Here's how the part is built. I have some questions about the finished solid (model axes, mm). A direction names the side the tool comes from. Give positions to 0.01 mm unless a question says otherwise; leave off trailing zeros. Order: outer loops, then holes, each group sorted by start corner. A loop starts at its lowest first (then second) coordinate and runs counter-clockwise, first axis right, second up. Notation, with made-up numbers: M 28,-27 L 74,-27 A20 ccw 74,12 Z; hole C 16,2 d2. An arc over 180 degrees is marked long. Use one line per item in the form item = value.
from build123d import *

# Parameters (mm, degrees)
SKETCH_1_W      = 50
SKETCH_1_H      = 50
SKETCH_1_R      = 13
SKETCH_1_R_2    = 2
EXTRUDE_1_DEPTH = 2
SKETCH_2_W      = 50
SKETCH_2_H      = 50
SKETCH_2_R      = 12.5
SKETCH_2_R_2    = 2.5
EXTRUDE_2_DEPTH = 2
EXTRUDE_3_DEPTH = 2


with BuildPart() as part:
    # 草图1 → 凸台-拉伸1 (new body)
    with BuildSketch(Plane(origin=(0, 0, 0), x_dir=(1, 0, 0), z_dir=(0, 1, 0))):
        Rectangle(SKETCH_1_W, SKETCH_1_H)
        with Locations(Location((0, 3, 0), (0, 0, 270))):
            Circle(SKETCH_1_R, mode=Mode.SUBTRACT)
        with Locations(Location((0, 20.5, 0), (0, 0, 270))):
            Circle(SKETCH_1_R_2, mode=Mode.SUBTRACT)
        with Locations(Location((0, -14.5, 0), (0, 0, 270))):
            Circle(SKETCH_1_R_2, mode=Mode.SUBTRACT)
        with Locations(Location((17.5, 3, 0), (0, 0, 270))):
            Circle(SKETCH_1_R_2, mode=Mode.SUBTRACT)
        with Locations(Location((-17.5, 3, 0), (0, 0, 270))):
            Circle(SKETCH_1_R_2, mode=Mode.SUBTRACT)
    extrude(amount=EXTRUDE_1_DEPTH)

    # 草图2 → 凸台-拉伸2 (add)
    with BuildSketch(Plane.XY.offset(25)):
        with Locations((0, 25)):
            Rectangle(SKETCH_2_W, SKETCH_2_H)
        with Locations((0, 26)):
            Circle(SKETCH_2_R, mode=Mode.SUBTRACT)
        with Locations((-15, 41)):
            Circle(SKETCH_2_R_2, mode=Mode.SUBTRACT)
        with Locations((15, 41)):
            Circle(SKETCH_2_R_2, mode=Mode.SUBTRACT)
        with Locations((15, 11)):
            Circle(SKETCH_2_R_2, mode=Mode.SUBTRACT)
        with Locations((-15, 11)):
            Circle(SKETCH_2_R_2, mode=Mode.SUBTRACT)
    extrude(amount=-EXTRUDE_2_DEPTH)

    # 草图3 → 凸台-拉伸3 (add)
    with BuildSketch(Plane(origin=(25, 0, 0), x_dir=(0, 0, -1), z_dir=(1, 0, 0))):
        Polygon((-25, 0), (0, 0), (-25, 25), align=None)
    extrude_3 = extrude(amount=-EXTRUDE_3_DEPTH)

    # 镜向2: 凸台-拉伸3 across plane
    add(extrude_3.mirror(Plane(origin=(0, 0, 0), x_dir=(0, 0, 1), z_dir=(1, 0, 0))))


solid = part.part
Q1. I want a section at C-C on y = 26. Write out the boundary of the cut face in (x, z), then the cut area to 3 significant figures.
Found:
outline = M -25,23 L -12.5,23 L -12.5,25 L -25,25 Z; M 12.5,23 L 25,23 L 25,25 L 12.5,25 Z
area = 50.0 mm²
Q2. I'm going to push flat-ended pins straight in: pin 1 Ø6 at (x, y) = (-15, 11) entering from -Z; pin 2 Ø2.5 at (x, z) = (0, 14.5) entering from +Y; pin 3 Ø1 at (x, z) = (19.5, 5) entering from +Y. Where does each tip first touch, or does it pass through?
Found:
pin_1 = 23
pin_2 = through
pin_3 = 2
Q3. Thinking about a two-plate mould opening in Z: for faces 1 (the face through (3.9, 1, 9.4)), 2 (the face through (24, 12, 12)), 3 (the face through (23, 8, 17)), which applies, +Z half, -Z half, draft (parallel to the pull), parting line (faces both ways), or undercut?
Found:
face_1 = undercut
face_2 = -Z half
face_3 = draft
Q4. I want a section at D-D on x = 0. Write out the boundary of the cut face in (y, z), then the cut area to 3 significant figures.
Found:
outline = M 0,-25 L 2,-25 L 2,-22.5 L 0,-22.5 Z; M 0,-18.5 L 2,-18.5 L 2,-16 L 0,-16 Z; M 0,10 L 2,10 L 2,12.5 L 0,12.5 Z; M 0,16.5 L 2,16.5 L 2,23 L 13.5,23 L 13.5,25 L 0,25 Z; M 38.5,23 L 50,23 L 50,25 L 38.5,25 Z
area = 78.0 mm²
Q5. I need wall thicknesses on L1, parallel to Y at x = -15, z = 24; L2, parallel to X at y = 8.5, z = 13; L3, parallel to Y at x = -10, z = -18.5. Which ranges of each line are inside material? Lowest first, please.
Found:
L1 = 0 to 8.5, 13.5 to 38.5, 43.5 to 50
L2 = -25 to -23, 23 to 25
L3 = 0 to 2
Q6. I want a section at B-B on y = 41. Write out the boundary of the cut face in (x, z).
Found:
outline = M -25,23 L -17.5,23 L -17.5,25 L -25,25 Z; M -12.5,23 L 12.5,23 L 12.5,25 L -12.5,25 Z; M 17.5,23 L 25,23 L 25,25 L 17.5,25 Z
Q7. I want a section at A-A on z = -20.5. Write out the boundary of the cut face in (x, y), then the cut area to 3 significant figures.
Found:
outline = M -25,0 L -2,0 L -2,2 L -25,2 Z; M 2,0 L 25,0 L 25,2 L 2,2 Z
area = 92.0 mm²
Q8. On a 3-axis mill with a long thin cutter (end or side, diameter ignored), from which of +Z, -Z, +X, -X, +Y, -Y can I reach the whole of each face in a straight line? I mean faces 4 (the face through (-11.5, 31.7, 23)), 5 (the face through (-15.517, 0.986, -3.26)). Say none if no direction works.
Found:
face_4 = -Z, +Y
face_5 = +Y, -Y
